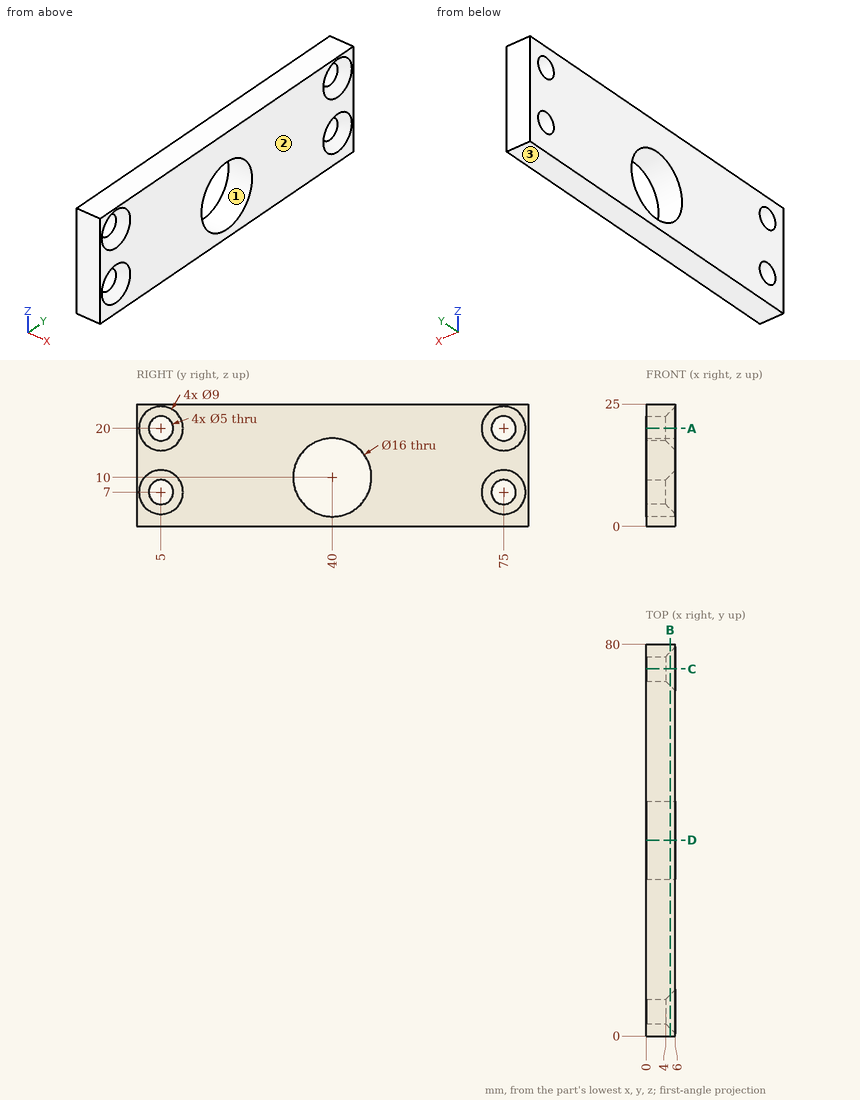
Geometry check sheet. Reference: drawing and pictorial views, mm from the part's lowest x, y, z. Round coordinates to 2 decimals unless told otherwise and drop trailing zeros. Order: outer loops, then holes, each group sorted by start corner. A loop starts at its lowest first (then second) coordinate and runs counter-clockwise, first axis right, second up. Notation, with made-up numbers: M -13.75,30 L 36.25,30 A24 ccw 36.25,69 Z; hole C -33,54 d5. An arc over 180 degrees is marked long. Answer in a Markdown table with one row per item.
(1) Sectioned sample at D-D, the plane y = 40. Record the cut outline in (x, z), and give its area (3 significant figures).
Responses:
| item | result |
|---|---|
| outline | M 0,0 L 6,0 L 6,2 L 0,2 Z; M 0,18 L 6,18 L 6,25 L 0,25 Z |
| area | 54.0 mm² |
(2) Scan lines: probe 1 along Y at (x, z) = (1.75, 20); probe 2 along Z at (x, y) = (1.65, 76.5); probe 3 along Y at (x, z) = (3.1, 7). Record each from-to range of solid material in increasing order. Write a range as from..to.
Responses:
| item | result |
|---|---|
| probe 1 | y = 0..2.5, 7.5..72.5, 77.5..80 |
| probe 2 | z = 0..5, 9..18, 22..25 |
| probe 3 | y = 0..2.5, 7.5..32.58, 47.42..72.5, 77.5..80 |
(3) Go/stop test with flat-tipped pins: P1, Ø4, axis at y = 75, z = 7, coming from the +X side; P2, Ø6, axis at y = 5, z = 7, coming from the +X side. Record where each tip stops, or that it passes through.
Responses:
| item | result |
|---|---|
| P1 | passes through |
| P2 | stops at x = 4.5 |
(4) Sectioned sample at A-A, the plane z = 20. Record the cut outline in (x, y).
Responses:
| item | result |
|---|---|
| outline | M 0,0 L 6,0 L 6,0.5 L 4,2.5 L 0,2.5 Z; M 0,7.5 L 4,7.5 L 6,9.5 L 6,70.5 L 4,72.5 L 0,72.5 Z; M 0,77.5 L 4,77.5 L 6,79.5 L 6,80 L 0,80 Z |
(5) Sectioned sample at B-B, the plane x = 4.9. Record the cut outline in (y, z).
Responses:
| item | result |
|---|---|
| outline | M 0,0 L 80,0 L 80,25 L 0,25 Z; hole C 5,7 d6.8; hole C 5,20 d6.8; hole C 40,10 d16; hole C 75,7 d6.8; hole C 75,20 d6.8 |
(6) Sectioned sample at C-C, the plane y = 75. Record the cut outline in (x, z), and give its area (3 significant figures).
Responses:
| item | result |
|---|---|
| outline | M 0,0 L 6,0 L 6,2.5 L 4,4.5 L 0,4.5 Z; M 0,9.5 L 4,9.5 L 6,11.5 L 6,15.5 L 4,17.5 L 0,17.5 Z; M 0,22.5 L 4,22.5 L 6,24.5 L 6,25 L 0,25 Z |
| area | 82.0 mm² |
(7) Draft check along Z on the marked faces 1, 2 and 3. Enter one of: released by +Z, released by -Z, zero draft, split by the parting line, or undercut.
Responses:
| item | result |
|---|---|
| face 1 | undercut |
| face 2 | zero draft |
| face 3 | released by -Z |
